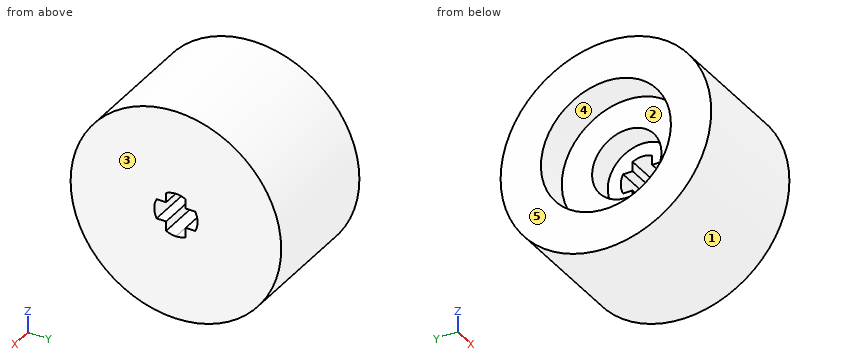
```python
from build123d import *

# Parameters (mm, degrees)
SKETCH_1_R          = 12.15
EXTRUDE_1_DEPTH     = 15
SKETCH_2_W          = 2.260059524
SKETCH_2_H          = 1.1
SKETCH_2_W_2        = 1.1
SKETCH_2_H_2        = 2.260059524
CUT_EXTRUDE_1_DEPTH = 23.80887985
SKETCH_3_R          = 7.5
CUT_EXTRUDE_2_DEPTH = 4
SKETCH_4_R          = 4
CUT_EXTRUDE_3_DEPTH = 3


with BuildPart() as part:
    # 草图1 → 凸台-拉伸1 (new body)
    with BuildSketch(Plane(origin=(0, 0, 0), x_dir=(0, 0, -1), z_dir=(1, 0, 0))):
        Circle(SKETCH_1_R)
    extrude(amount=EXTRUDE_1_DEPTH)

    # 草图2 → 切除-拉伸1 (cut, through all)
    with BuildSketch(Plane(origin=(15, 0, 0), x_dir=(0, 0, -1), z_dir=(1, 0, 0))):
        with Locations((0, 1.680029762)):
            Rectangle(SKETCH_2_W, SKETCH_2_H)
        with Locations((-1.680029762, 0)):
            Rectangle(SKETCH_2_W_2, SKETCH_2_H_2)
        with Locations((0, -1.680029762)):
            Rectangle(SKETCH_2_W, SKETCH_2_H)
        with Locations((1.680029762, 0)):
            Rectangle(SKETCH_2_W_2, SKETCH_2_H_2)
        Rectangle(SKETCH_2_W, SKETCH_2_H_2)
        with BuildLine():
            ThreePointArc((1.130029762, 2.230029762), (0, 2.5), (-1.130029762, 2.230029762))
            Line((-1.130029762, 2.230029762), (1.130029762, 2.230029762))
        make_face()
        with BuildLine():
            ThreePointArc((2.5, 0), (2.431570933, 0.580915483), (2.230029762, 1.130029762))
            Line((2.230029762, 1.130029762), (2.230029762, -1.130029762))
            ThreePointArc((2.230029762, -1.130029762), (2.431570933, -0.580915483), (2.5, 0))
        make_face()
        with BuildLine():
            Line((1.130029762, -2.230029762), (-1.130029762, -2.230029762))
            ThreePointArc((-1.130029762, -2.230029762), (0, -2.5), (1.130029762, -2.230029762))
        make_face()
        with BuildLine():
            Line((-2.230029762, -1.130029762), (-2.230029762, 1.130029762))
            ThreePointArc((-2.230029762, 1.130029762), (-2.5, 0), (-2.230029762, -1.130029762))
        make_face()
    extrude(amount=-CUT_EXTRUDE_1_DEPTH, mode=Mode.SUBTRACT)

    # 草图3 → 切除-拉伸2 (cut)
    with BuildSketch(Plane.ZY):
        Circle(SKETCH_3_R)
    extrude(amount=-CUT_EXTRUDE_2_DEPTH, mode=Mode.SUBTRACT)

    # 草图4 → 切除-拉伸3 (cut)
    with BuildSketch(Plane.ZY.offset(-4)):
        Circle(SKETCH_4_R)
    extrude(amount=-CUT_EXTRUDE_3_DEPTH, mode=Mode.SUBTRACT)


solid = part.part
```
CAD build for the part. Positions are in the model's coordinates, mm. Face numbers are marked on the shaded views. A direction names the side the tool comes from. Give positions to 0.01 mm unless a question says otherwise; leave off trailing zeros. Loops run counter-clockwise (first coordinate to the right, second up) from the corner with the lowest first, then second, coordinate; pieces in that order, holes last. Notation, with made-up numbers: M 0,83.5 L 39,83.5 A26 ccw 39,120.5 Z; hole C 17.5,-30.75 d9. An arc over 180 degrees is marked long. Use one line per item in the form item = value.
Item 1: Slice it at A-A (z = 0). List the corners of the cut face in (x, y).
Determined:
outline = M 0,-12.15 L 15,-12.15 L 15,-2.5 L 7,-2.5 L 7,-4 L 4,-4 L 4,-7.5 L 0,-7.5 Z; M 0,7.5 L 4,7.5 L 4,4 L 7,4 L 7,2.5 L 15,2.5 L 15,12.15 L 0,12.15 Z
Item 2: Which spindle directions (+Z, -Z, +X, -X, +Y, -Y) get a long thin tool onto all of the face, cutting with end or side? Do the marked faces 4 and 5. Say none if no direction does.
Determined:
face_4 = -X
face_5 = +Z, -Z, -X, +Y, -Y
Item 3: Slice it at B-B (x = 9). List the corners of the cut face in (y, z), plus the area to 3 significant figures.
Determined:
outline = C 0,0 d24.3; hole M -2.23,-1.13 L -1.13,-1.13 L -1.13,-2.23 A2.5 ccw 1.13,-2.23 L 1.13,-1.13 L 2.23,-1.13 A2.5 ccw 2.23,1.13 L 1.13,1.13 L 1.13,2.23 A2.5 ccw -1.13,2.23 L -1.13,1.13 L -2.23,1.13 A2.5 ccw Z
area = 447 mm2
Item 4: Flat gauge pins, fed straight in: pin 1 (1.2 mm diameter, centred on x = 12.5, z = 1.5, fed in from -Y); pin 2 (0.9 mm diameter, centred on x = 11.5, y = 2, fed in from +Z); pin 3 (4 mm diameter, centred on x = 3.5, y = 2, fed in from -Z); pin 4 (9 mm diameter, centred on y = -0.5, z = 1.5, fed in from -X). Where does each tip first touch, or does it go through?
Determined:
pin_1 = -12.12
pin_2 = 12.05
pin_3 = -12.15
pin_4 = 4
Item 5: Slice it at C-C (y = -1.5). List the corners of the cut face in (x, z), plus the area to 3 significant figures.
Determined:
outline = M 0,-12.06 L 15,-12.06 L 15,-1.13 L 7,-1.13 L 7,-3.71 L 4,-3.71 L 4,-7.35 L 0,-7.35 Z; M 0,7.35 L 4,7.35 L 4,3.71 L 7,3.71 L 7,1.13 L 15,1.13 L 15,12.06 L 0,12.06 Z
area = 263 mm2
Item 6: Two-plate mould, pull along Y, no slides. Class the marked faces 1, 2 and 3: pulls with the +Y half, pulls with the -Y half, needs draft (parallel to the pull), parting line crosses it, or undercut.
Determined:
face_1 = parting line crosses it
face_2 = undercut
face_3 = needs draft
Item 7: Slice it at D-D (z = 3.25). List the corners of the cut face in (x, y), plus the area to 3 significant figures.
Determined:
outline = M 0,-11.71 L 15,-11.71 L 15,11.71 L 0,11.71 L 0,6.76 L 4,6.76 L 4,2.33 L 7,2.33 L 7,-2.33 L 4,-2.33 L 4,-6.76 L 0,-6.76 Z
area = 283 mm2
Item 8: Drill centre lines: probe 1 along Y at (x, z) = (5.25, 0); probe 2 along Y at (x, z) = (1.6, 0); probe 3 along X at (y, z) = (-4, -3.5). Where is each one in solid material? Low to high. Write a range as from..to.
Determined:
probe_1 = -12.15..-4, 4..12.15
probe_2 = -12.15..-7.5, 7.5..12.15
probe_3 = 4..15
